Autodesk Inventor part; units mm, degrees
sketch "スケッチ1" plane through (0, 0, 0) normal (0, 0, 1) x (1, 0, 0)
  circle A0 centre (0, 0) radius 117
  arc A1 (-7, 24) -> (7, 24) centre (0, 0) ccw
  line L0 (0, 25) -> (0, 28.8)
  line L1 (0, 28.8) -> (0, 20)
  line L2 (0, 20) -> (-7, 20)
  line L3 (-7, 24) -> (-7, 28.8)
  line L4 (-7, 28.8) -> (7, 28.8)
  line L5 (7, 28.8) -> (7, 24)
  line L6 (7, 20) -> (0, 20)
  circle A2 centre (0, 0) radius 111 construction
  circle A3 centre (0, 0) radius 103.5 construction
  circle A4 centre (0, 0) radius 104.3059 construction
  dimension "d0" = 234
  dimension "d1" = 50
  dimension "d2" = 3.8
  dimension "d3" = 8.8
  dimension "d4" = 7
  dimension "d5" = 14
  dimension "d8" = 222
  dimension "d9" = 207
  dimension "d10" = 208.6117
extrude "押し出し1" add sketch "スケッチ1" along normal blind 60
properties part number "gear4"
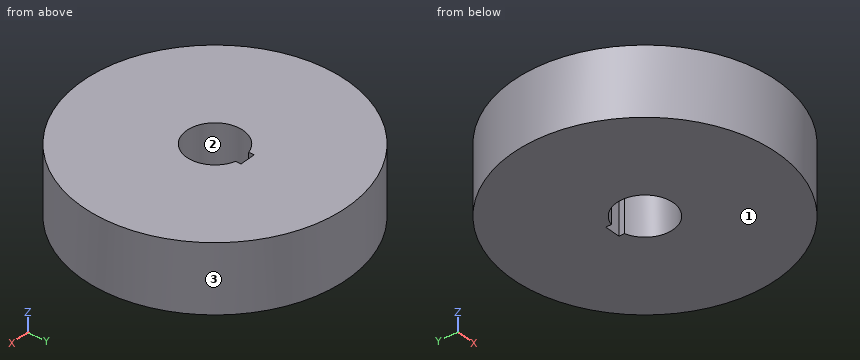
CAD build for the part. Positions are in the model's coordinates, mm. Face numbers are marked on the shaded views. Round coordinates to 2 decimals unless told otherwise and drop trailing zeros. Write each loop counter-clockwise with the first axis right and the second up, starting at its lowest first coordinate (ties: lowest second). Pieces come first, ordered by that corner, then holes.
(1) Mould opens along Y. For the marked faces 1, 2 and 3 say: pulls with the +Y half, pulls with the -Y half, needs draft (parallel to the pull), parting line crosses it, or undercut.
(2) Probe line 1 along Y through (x, z) = (0, 34.5); line 2 along X through (y, z) = (25.5, 50.5); line 3 along Y through (x, z) = (-13, 38). List the from-to ranges inside material, lowest first.
(3) Drop flat-ended pins along their axis: P1, Ø2, axis at x = 34, z = 10, coming from the -Y side; P2, Ø1.4, axis at y = 27.5, z = 34.5, coming from the +X side; P3, Ø10, axis at x = -54.5, z = 39, coming from the +Y side. Give the stop position or say it passes through.
(4) Slice it at A-A, the plane y = 0. Write the cut outline in (x, z), and give its area (3 significant figures).
(5) Slice it at C-C, the plane z = 7. Write the cut outline in (x, y), and give its area (3 significant figures).
(6) Slice it at D-D, the plane x = 51. Write the cut outline in (y, z), and give its area (3 significant figures).
(7) Slice it at B-B, the plane x = 0. Write the cut outline in (y, z), and give its area (3 significant figures).
From the geometry:
1. face 1: needs draft
1. face 2: undercut
1. face 3: parting line crosses it
2. line 1: y = -117 to -25, 28.8 to 117
2. line 2: x = -114.19 to -7, 7 to 114.19
2. line 3: y = -116.28 to -21.35, 21.35 to 116.28
3. P1: stops at y = -112.25
3. P2: stops at x = 113.89
3. P3: stops at y = 106.01
4. outline: (-117, 0) - (-25, 0) - (-25, 60) - (-117, 60) - close; (25, 0) - (117, 0) - (117, 60) - (25, 60) - close
4. area: 11,000 mm2
5. outline: circle Ø234 at (0, 0); hole (-7, 24) arc R25 ccw (long way) to (7, 24) - (7, 28.8) - (-7, 28.8) - close
5. area: 41,000 mm2
6. outline: (-105.3, 0) - (105.3, 0) - (105.3, 60) - (-105.3, 60) - close
6. area: 12,600 mm2
7. outline: (-117, 0) - (-25, 0) - (-25, 60) - (-117, 60) - close; (28.8, 0) - (117, 0) - (117, 60) - (28.8, 60) - close
7. area: 10,800 mm2
